```python
from build123d import *

# Parameters (mm, degrees)
F7_R     = 25.4
F8_DEPTH = 520.7
F6_R     = 25.4
F9_DEPTH = 520.7


with BuildPart() as f8:
    # F7 (on offset) → F8 (new body, through all)
    with BuildSketch(Plane.YZ.offset(520.7)):
        Circle(F7_R)
    extrude(amount=-F8_DEPTH)



with BuildPart() as f8b:
    # F7 (on offset) → F8, piece 2 (new body, through all)
    with BuildSketch(Plane.YZ.offset(520.7)):
        with Locations((0, 292.1)):
            Circle(F7_R)
    extrude(amount=-F8_DEPTH)


with BuildPart() as f8_1:
    add(f8.part)

    add(f8b.part)  # F9 merges F8b
    # F6 (on offset) → F9 (join, through all)
    with BuildSketch(Plane.XY.offset(520.7)):
        Circle(F6_R)
        with Locations((292.1, 0)):
            Circle(F6_R)
    extrude(amount=-F9_DEPTH)


solid = f8_1.part
```
Here's how the part is built. I have some questions about the finished solid (model axes, mm). A direction names the side the tool comes from. Round coordinates to 2 decimals unless told otherwise and drop trailing zeros. Write each loop counter-clockwise with the first axis right and the second up, starting at its lowest first coordinate (ties: lowest second). Pieces come first, ordered by that corner, then holes.
Q1. If we section it at C-C on z = 143: Write out the boundary of the cut face in (x, y), plus the area to 3 significant figures.
Q2. If we section it at A-A on y = 0: Write out the boundary of the cut face in (x, z).
Q3. If we section it at D-D on z = 14: Write out the boundary of the cut face in (x, y).
Q4. Please list where these lines run through material, in increasing order: probe 1 along Z at (x, y) = (385, 2); probe 2 along Z at (x, y) = (128.5, 12.5).
Q5. If we section it at B-B on x = 175: Write out the boundary of the cut face in (y, z), plus the area to 3 significant figures.
Q6. If we mould it in two halves opening along X, with no side actions, what happens to faces 1 (the flat face through (520.7, 0, 0)), 2 (the cylindrical face through (263.995, 24.227, 7.629)), 3 (the cylindrical face through (408, 23.463, 282.372))? For each: +X half, -X half, draft (parallel to the pull), parting line (faces both ways), or undercut.
Q7. Will these pins go through, and if not, where does the flat tip stop? P1, Ø4, axis at x = 136, y = 13, coming from the +Z side; P2, Ø4, axis at x = 418, y = 10, coming from the -Z side; P3, Ø12.5, axis at x = -6.5, y = 3.5, coming from the -Z side.
Q8. Which directions (+Z, -Z, +X, -X, +Y, -Y) give clear straight access to the entire face, cutting with the end or side of a thin tool? Please do faces 4 (the cylindrical face through (316.327, 7.629, 408)), 5 (the flat face through (-10, 0, 0)), 6 (the cylindrical face through (148.095, 23.463, 282.372)).
Answer below:
1. outline: circle Ø50.8 at (0, 0); circle Ø50.8 at (292.1, 0)
1. area: 4,050 mm2
2. outline: (-25.4, 0) - (0, 0) - (0, -25.4) - (520.7, -25.4) - (520.7, 25.4) - (317.5, 25.4) - (317.5, 266.7) - (520.7, 266.7) - (520.7, 317.5) - (317.5, 317.5) - (317.5, 520.7) - (266.7, 520.7) - (266.7, 317.5) - (25.4, 317.5) - (25.4, 520.7) - (-25.4, 520.7) - close; hole (25.4, 25.4) - (266.7, 25.4) - (266.7, 266.7) - (25.4, 266.7) - close
3. outline: (14, -21.19) - (278.1, -21.19) arc R25.4 ccw to (306.1, -21.19) - (520.7, -21.19) - (520.7, 21.19) - (306.1, 21.19) arc R25.4 ccw to (278.1, 21.19) - (14, 21.19) arc R25.4 ccw (long way) to start
4. probe 1: z = -25.32 to 25.32, 266.78 to 317.42
4. probe 2: z = -22.11 to 22.11, 269.99 to 314.21
5. outline: circle Ø50.8 at (0, 0); circle Ø50.8 at (0, 292.1)
5. area: 4,050 mm2
6. face 1: +X half
6. face 2: undercut
6. face 3: draft
7. P1: stops at z = 314.99
7. P2: stops at z = -24.11
7. P3: stops at z = 0
8. face 4: +Z
8. face 5: -Z, -X, +Y, -Y
8. face 6: none
